Verification items for the finished model (mm, model axes). A direction names the side the tool comes from. Round coordinates to 2 decimals unless told otherwise and drop trailing zeros. Loops run counter-clockwise (first coordinate to the right, second up) from the corner with the lowest first, then second, coordinate; pieces in that order, holes last.
from build123d import *

# Parameters (mm, degrees)
FILLET1_R = 0.254


with BuildPart() as part:
    # Sketch1 → Revolve1 (revolve)
    with BuildSketch(Plane(origin=(0, 0, 0), x_dir=(1, 0, 0), z_dir=(0, 1, 0))):
        Polygon((5.126280771, 31.75), (4.8514, 0), (4.8387, 0), (5.124663893, -33.02), (7.970733756, -33.02), (8.5471, 0), (8.5598, 0), (8.005601689, 31.75), align=None)
    revolve(axis=Axis((0, 0, -31.75297092), (0, 0, 1)))

    # Fillet1
    fillet1_edges = [part.edges().sort_by_distance(p)[0] for p in [
        (-8.005601689, 0, -31.75),
        (-7.970733756, 0, 33.02),
        (-5.124663893, 0, 33.02),
        (-5.126280771, 0, -31.75),
    ]]
    fillet(fillet1_edges, radius=FILLET1_R)


solid = part.part
1. Section check A-A (z = -4.5). Enter the section's corners in (x, y), then the cut area to 3 significant figures.
2. Scan lines: L1, parallel to X at y = 4, z = -7; L2, parallel to X at y = 3.75, z = -12; L3, parallel to Y at x = 0.5, z = -10. Record each from-to range of solid material in increasing order.
3. Tool access check on faces 1 (the face through (5.3, -1.6, 33.02)), 2 (the face through (4.756, 1.498, -15.529)), 3 (the face through (7.883, 2.483, 16.156)). Record the directions out of +Z, -Z, +X, -X, +Y, -Y that give a thin tool (end or side, any length) a straight path to the whole face; none if there is none.
4. Gauge pin test, flat ends, axial feed: P1, Ø3, axis at y = 4, z = 5, coming from the -X side; P2, Ø5, axis at x = 0, y = -3.5, coming from the +Z side; P3, Ø8, axis at x = -3.5, z = 12.5, coming from the +Y side; P4, Ø10, axis at x = -5.5, z = -20.5, coming from the +Y side. Record the tip position at first contact, or that the pin passes through.
5. Release check for a two-part mould opening along X. For faces 4 (the face through (-3.954, -3.032, 16.613)), 5 (the face through (-8.273, 0.364, -15.971)), 6 (the face through (1.6, 5.3, -31.75)) record: released by +X, released by -X, zero draft, split by the parting line, or undercut.
6. Section check B-B (z = 6.5). Enter the section's corners in (x, y) (3 decimals), then the cut area to 3 significant figures.
Taken from the geometry:
1. outline: circle Ø16.96 at (0, 0); hole circle Ø9.78 at (0, 0)
1. area: 151 mm2
2. L1: x = -7.43 to -2.85, 2.85 to 7.43
2. L2: x = -7.46 to -3.24, 3.24 to 7.46
2. L3: y = -8.37 to -4.91, 4.91 to 8.37
3. face 1: +Z, +X, -X, +Y, -Y
3. face 2: -Z
3. face 3: +Z
4. P1: stops at x = -8.08
4. P2: stops at z = 33.02
4. P3: stops at y = 8.37
4. P4: stops at y = 8.2
5. face 4: undercut
5. face 5: split by the parting line
5. face 6: zero draft
6. outline: circle Ø16.867 at (0, 0); hole circle Ø9.79 at (0, 0)
6. area: 148 mm2
